```python
from build123d import *

# Parameters (mm, degrees)
F0_W          = 140
F0_H          = 60
F1_DEPTH      = 60
F2_R          = 10
F5_DEPTH      = 20
F4_R          = 10
F6_DEPTH      = 71.6
F3_R          = 10
F7_DEPTH      = 10
F8_R          = 5
F9_T1_DEPTH   = 165
F9_T3_DEPTH   = 67.5
F9_S7_W       = 5
F9_S7_H       = 5
F9_T8_DEPTH   = 5
F10_T1_DEPTH  = 50
F10_T3_DEPTH  = 67.5
F10_S7_W      = 5
F10_S7_H      = 5
F10_T8_DEPTH  = 5
F10_T12_ANGLE = 89.9999999974
F11_T1_DEPTH  = 147.5
F11_T3_DEPTH  = 50
F11_S7_W      = 5
F11_S7_H      = 5
F11_T8_DEPTH  = 5
F11_T12_ANGLE = 89.9999999974
F12_T1_DEPTH  = 50
F12_T3_DEPTH  = 50
F12_S7_W      = 5
F12_S7_H      = 5
F12_T8_DEPTH  = 5
F12_S13_W     = 5
F12_S13_H     = 5
F12_T14_DEPTH = 5
F12_T18_ANGLE = 89.9999999974


# Not quite as in the source:
# - a fillet or chamfer that OpenCascade refuses, or shapes differently, is made with other operations: its cross-section is extruded or revolved along the edge and cut away or added


with BuildPart() as f1:
    # F0 (on Top) → F1 (new body)
    with BuildSketch(Plane.XY):
        Rectangle(F0_W, F0_H)
    extrude(amount=F1_DEPTH)

    # F2 (on face) → F5 (join)
    with BuildSketch(Plane.XY.offset(60)):
        with Locations((-40, 0)):
            Circle(F2_R)
    extrude(amount=F5_DEPTH)

    # F4 (on face) → F6 (cut)
    with BuildSketch(Plane.XY.offset(60)):
        Circle(F4_R)
    extrude(amount=-F6_DEPTH, mode=Mode.SUBTRACT)

    # F3 (on face) → F7 (cut)
    with BuildSketch(Plane.XY.offset(60)):
        with Locations((40, 0)):
            Circle(F3_R)
    extrude(amount=-F7_DEPTH, mode=Mode.SUBTRACT)

    # F8
    f8_edges = [f1.edges().sort_by_distance(p)[0] for p in [
        (0, 30, 60),
        (-70, 0, 60),
        (0, -30, 60),
        (70, 0, 60),
    ]]
    fillet(f8_edges, radius=F8_R)

    # F9: fillet of radius 5 on 2 edges, made by hand

    # F9_s2 → F9_t1 (cut)
    with BuildSketch(Plane.YZ.offset(-82.5)):
        with BuildLine():
            ThreePointArc((-30, 5), (-28.5355339059, 1.4644660941), (-25, 0))
            Line((-25, 0), (-30, 0))
            Line((-30, 0), (-30, 5))
        make_face()
    extrude(amount=F9_T1_DEPTH, mode=Mode.SUBTRACT)

    # F9_s4 → F9_t3 (cut)
    with BuildSketch(Plane.XY.offset(-12.5)):
        with BuildLine():
            ThreePointArc((65, -30), (68.5355339059, -28.5355339059), (70, -25))
            Line((70, -25), (70, -30))
            Line((70, -30), (65, -30))
        make_face()
    extrude(amount=F9_T3_DEPTH, mode=Mode.SUBTRACT)


with BuildPart() as f9_tool6:
    # F9_s7 → F9_t8 (new body)
    with BuildSketch(Plane.XZ.offset(25)):
        with Locations((67.5, 57.5)):
            Rectangle(F9_S7_W, F9_S7_H)
    extrude(amount=F9_T8_DEPTH)

    # F9_s9 → F9_t10 (revolve, cut)
    with BuildSketch(Plane(origin=(65, -25, 55), x_dir=(-0.7071067812, 0, -0.7071067812), z_dir=(-0.7071067812, 0, 0.7071067812))):
        with BuildLine():
            ThreePointArc((0, -5), (5, 0), (0, 5))
            Line((0, 5), (0, -5))
        make_face()
    revolve(axis=Axis((65, -25, 55), (0, -1, 0)), mode=Mode.SUBTRACT)


with BuildPart() as f1_1:
    add(f1.part)

    # F9_t5: cut F9_tool6
    add(f9_tool6.part, mode=Mode.SUBTRACT)

    # F10: fillet of radius 5 on 1 edges, made by hand

    # F10_s2 → F10_t1 (cut)
    with BuildSketch(Plane.XY.offset(5)):
        with BuildLine():
            ThreePointArc((-65, -30), (-68.5355339059, -28.5355339059), (-70, -25))
            Line((-70, -25), (-70, -30))
            Line((-70, -30), (-65, -30))
        make_face()
    extrude(amount=F10_T1_DEPTH, mode=Mode.SUBTRACT)

    # F10_s4 → F10_t3 (cut)
    with BuildSketch(Plane.XZ.offset(-42.5)):
        with BuildLine():
            ThreePointArc((-70, 5), (-68.5355339059, 1.4644660941), (-65, 0))
            Line((-65, 0), (-70, 0))
            Line((-70, 0), (-70, 5))
        make_face()
    extrude(amount=F10_T3_DEPTH, mode=Mode.SUBTRACT)


with BuildPart() as f10_tool6:
    # F10_s7 → F10_t8 (new body)
    with BuildSketch(Plane.XZ.offset(25)):
        with Locations((-67.5, 57.5)):
            Rectangle(F10_S7_W, F10_S7_H)
    extrude(amount=F10_T8_DEPTH)

    # F10_s9 → F10_t10 (revolve, cut)
    with BuildSketch(Plane(origin=(-65, -25, 55), x_dir=(0.7071067812, 0, -0.7071067812), z_dir=(-0.7071067812, 0, -0.7071067812))):
        with BuildLine():
            ThreePointArc((0, -5), (5, 0), (0, 5))
            Line((0, 5), (0, -5))
        make_face()
    revolve(axis=Axis((-65, -25, 55), (0, -1, 0)), mode=Mode.SUBTRACT)


with BuildPart() as f1_2:
    add(f1_1.part)

    # F10_t5: cut F10_tool6
    add(f10_tool6.part, mode=Mode.SUBTRACT)

    # F10_s11 → F10_t12 (revolve, cut)
    with BuildSketch(Plane.XZ.offset(24.9999999999)):
        with BuildLine():
            ThreePointArc((-65, 0), (-68.5355339059, 1.4644660941), (-70, 5))
            Line((-70, 5), (-70, 0))
            Line((-70, 0), (-65, 0))
        make_face()
    revolve(axis=Axis((-70, -24.9999999999, 5.0000000001), (-1, 0, 0)), revolution_arc=F10_T12_ANGLE, mode=Mode.SUBTRACT)

    # F11: fillet of radius 5 on 1 edges, made by hand

    # F11_s2 → F11_t1 (cut)
    with BuildSketch(Plane.YZ.offset(-65)):
        with BuildLine():
            ThreePointArc((25, 0), (28.5355339059, 1.4644660941), (30, 5))
            Line((30, 5), (30, 0))
            Line((30, 0), (25, 0))
        make_face()
    extrude(amount=F11_T1_DEPTH, mode=Mode.SUBTRACT)

    # F11_s4 → F11_t3 (cut)
    with BuildSketch(Plane.XY.offset(5)):
        with BuildLine():
            ThreePointArc((-65, 30), (-68.5355339059, 28.5355339059), (-70, 25))
            Line((-70, 25), (-70, 30))
            Line((-70, 30), (-65, 30))
        make_face()
    extrude(amount=F11_T3_DEPTH, mode=Mode.SUBTRACT)


with BuildPart() as f11_tool6:
    # F11_s7 → F11_t8 (new body)
    with BuildSketch(Plane.XZ.offset(-25)):
        with Locations((-67.5, 57.5)):
            Rectangle(F11_S7_W, F11_S7_H)
    extrude(amount=-F11_T8_DEPTH)

    # F11_s9 → F11_t10 (revolve, cut)
    with BuildSketch(Plane(origin=(-65, 25, 55), x_dir=(0.7071067812, 0, -0.7071067812), z_dir=(0.7071067812, 0, 0.7071067812))):
        with BuildLine():
            ThreePointArc((0, -5), (5, 0), (0, 5))
            Line((0, 5), (0, -5))
        make_face()
    revolve(axis=Axis((-65, 25, 55), (0, 1, 0)), mode=Mode.SUBTRACT)


with BuildPart() as f1_3:
    add(f1_2.part)

    # F11_t5: cut F11_tool6
    add(f11_tool6.part, mode=Mode.SUBTRACT)

    # F11_s11 → F11_t12 (revolve, cut)
    with BuildSketch(Plane.YZ.offset(-64.9999999999)):
        with BuildLine():
            ThreePointArc((30, 5), (28.5355339059, 1.4644660941), (25, 0))
            Line((25, 0), (30, 0))
            Line((30, 0), (30, 5))
        make_face()
    revolve(axis=Axis((-64.9999999999, 30, 5.0000000001), (0, 1, 0)), revolution_arc=F11_T12_ANGLE, mode=Mode.SUBTRACT)

    # F12: fillet of radius 5 on 1 edges, made by hand

    # F12_s2 → F12_t1 (cut)
    with BuildSketch(Plane.XY.offset(5)):
        with BuildLine():
            ThreePointArc((70, 25), (68.5355339059, 28.5355339059), (65, 30))
            Line((65, 30), (70, 30))
            Line((70, 30), (70, 25))
        make_face()
    extrude(amount=F12_T1_DEPTH, mode=Mode.SUBTRACT)

    # F12_s4 → F12_t3 (cut)
    with BuildSketch(Plane.XZ.offset(-25)):
        with BuildLine():
            ThreePointArc((65, 0), (68.5355339059, 1.4644660941), (70, 5))
            Line((70, 5), (70, 0))
            Line((70, 0), (65, 0))
        make_face()
    extrude(amount=F12_T3_DEPTH, mode=Mode.SUBTRACT)


with BuildPart() as f12_tool6:
    # F12_s7 → F12_t8 (new body)
    with BuildSketch(Plane.YZ.offset(65)):
        with Locations((27.5, 57.5)):
            Rectangle(F12_S7_W, F12_S7_H)
    extrude(amount=F12_T8_DEPTH)

    # F12_s9 → F12_t10 (revolve, cut)
    with BuildSketch(Plane(origin=(65, 25, 55), x_dir=(0, -0.7071067812, -0.7071067812), z_dir=(0, -0.7071067812, 0.7071067812))):
        with BuildLine():
            ThreePointArc((0, -5), (5, 0), (0, 5))
            Line((0, 5), (0, -5))
        make_face()
    revolve(axis=Axis((65, 25, 55), (1, 0, 0)), mode=Mode.SUBTRACT)


with BuildPart() as f1_4:
    add(f1_3.part)

    # F12_t5: cut F12_tool6
    add(f12_tool6.part, mode=Mode.SUBTRACT)


with BuildPart() as f12_tool12:
    # F12_s13 → F12_t14 (new body)
    with BuildSketch(Plane.XY.offset(5)):
        with Locations((67.5, -27.5)):
            Rectangle(F12_S13_W, F12_S13_H)
    extrude(amount=-F12_T14_DEPTH)

    # F12_s15 → F12_t16 (revolve, cut)
    with BuildSketch(Plane(origin=(65, -25, 5), x_dir=(-0.7071067812, 0.7071067812, 0), z_dir=(-0.7071067812, -0.7071067812, 0))):
        with BuildLine():
            ThreePointArc((0, -5), (5, 0), (0, 5))
            Line((0, 5), (0, -5))
        make_face()
    revolve(axis=Axis((65, -25, 5), (0, 0, -1)), mode=Mode.SUBTRACT)


with BuildPart() as f1_5:
    add(f1_4.part)

    # F12_t11: cut F12_tool12
    add(f12_tool12.part, mode=Mode.SUBTRACT)

    # F12_s17 → F12_t18 (revolve, cut)
    with BuildSketch(Plane.XY.offset(5.0000000001)):
        with BuildLine():
            ThreePointArc((70, 25), (68.5355339059, 28.5355339059), (65, 30))
            Line((65, 30), (70, 30))
            Line((70, 30), (70, 25))
        make_face()
    revolve(axis=Axis((70, 24.9999999999, 5.0000000001), (-1, 0, 0)), revolution_arc=F12_T18_ANGLE, mode=Mode.SUBTRACT)


solid = f1_5.part
```
Can you work these out from the model? Positions are in its coordinate system, mm. A direction names the side the tool comes from. Give positions to 0.01 mm unless a question says otherwise; leave off trailing zeros. Order: outer loops, then holes, each group sorted by start corner. A loop starts at its lowest first (then second) coordinate and runs counter-clockwise, first axis right, second up. Notation, with made-up numbers: (-2, 35.25) - (19, 35.25) arc R34 ccw to (19, 72.25) - close; hole circle Ø10 at (88.25, 73.5). An arc over 180 degrees is marked (long way). Use a Markdown table: item, result. Add a question column.
Q1. If we section it at B-B on z = 30: Write out the boundary of the cut face in (x, y), plus the area to 3 significant figures.
Q2. Please list where these lines run through material, in increasing order: line 1 along Y through (x, z) = (40, 53.5); line 2 along Z through (x, y) = (-8, -14.5); line 3 along Y through (x, z) = (8, 54).
Q3. If we section it at C-C on x = 0: Write out the boundary of the cut face in (y, z), plus the area to 3 significant figures.
Q4. If we section it at A-A on y = -6: Write out the boundary of the cut face in (x, z).
Q5. If we mould it in two halves opening along Y, with no side actions, what happens to faces 3 (the cylindrical face through (-1, 28, 1)), 4 (the cylindrical face through (-1, -29, 2)), 5 (the cylindrical face through (-2.17, -9.76, 30.42))? For each: released by +Y, released by -Y, zero draft, split by the parting line, or undercut.
Q6. I'm going to push flat-ended pins straight in: pin 1 (3 mm diameter, centred on x = -44.5, y = -11.5, fed in from +Z); pin 2 (12 mm diameter, centred on x = 40, y = 0, fed in from +Z); pin 3 (8 mm diameter, centred on y = 19.5, z = 65, fed in from +X). Where does each tip first touch, or does it pass through?
Q7. On a 3-axis mill with a long thin cutter (end or side, diameter ignored), from which of +Z, -Z, +X, -X, +Y, -Y can I reach the whole of each face in a straight line? I mean faces 1 (the flat face through (70, 0, 30)), 2 (the cylindrical face through (-50, 0, 70)). Say none if no direction works.
Q8. If we section it at D-D on y = 20: Write out the boundary of the cut face in (x, z).
Answers follow:
| question | item | result |
|---|---|---|
| 1 | outline | (-70, -25) arc R5 ccw to (-65, -30) - (65, -30) arc R5 ccw to (70, -25) - (70, 25) arc R5 ccw to (65, 30) - (-65, 30) arc R5 ccw to (-70, 25) - close; hole circle Ø20 at (0, 0) |
| 1 | area | 8,060 mm^2 |
| 2 | line 1 | y = -30 to -10, 10 to 30 |
| 2 | line 2 | z = 0 to 60 |
| 2 | line 3 | y = -30 to -6, 6 to 30 |
| 3 | outline | (-30, 5) arc R5 ccw to (-25, 0) - (-10, 0) - (-10, 60) - (-25, 60) arc R5 ccw to (-30, 55) - close; (10, 0) - (25, 0) arc R5 ccw to (30, 5) - (30, 55) arc R5 ccw to (25, 60) - (10, 60) - close |
| 3 | area | 2,380 mm^2 |
| 4 | outline | (-70, 5) arc R5 ccw to (-65, 0) - (-8, 0) - (-8, 60) - (-32, 60) - (-32, 80) - (-48, 80) - (-48, 60) - (-65, 60) arc R5 ccw to (-70, 55) - close; (8, 0) - (65, 0) arc R5 ccw to (70, 5) - (70, 55) arc R5 ccw to (65, 60) - (48, 60) - (48, 50) - (32, 50) - (32, 60) - (8, 60) - close |
| 5 | face 3 | released by +Y |
| 5 | face 4 | released by -Y |
| 5 | face 5 | undercut |
| 6 | pin 1 | stops at z = 60 |
| 6 | pin 2 | stops at z = 50 |
| 6 | pin 3 | passes through |
| 7 | face 1 | +Z, -Z, +X, +Y, -Y |
| 7 | face 2 | +Z |
| 8 | outline | (-70, 5) arc R5 ccw to (-65, 0) - (65, 0) arc R5 ccw to (70, 5) - (70, 55) arc R5 ccw to (65, 60) - (-65, 60) arc R5 ccw to (-70, 55) - close |
